Part print with two shaded views. Sizes in mm from the minimum x, y, z corner. A direction names the side the tool comes from. Give positions to 0.01 mm unless a question says otherwise; leave off trailing zeros. Write each loop counter-clockwise with the first axis right and the second up, starting at its lowest first coordinate (ties: lowest second). Pieces come first, ordered by that corner, then holes.
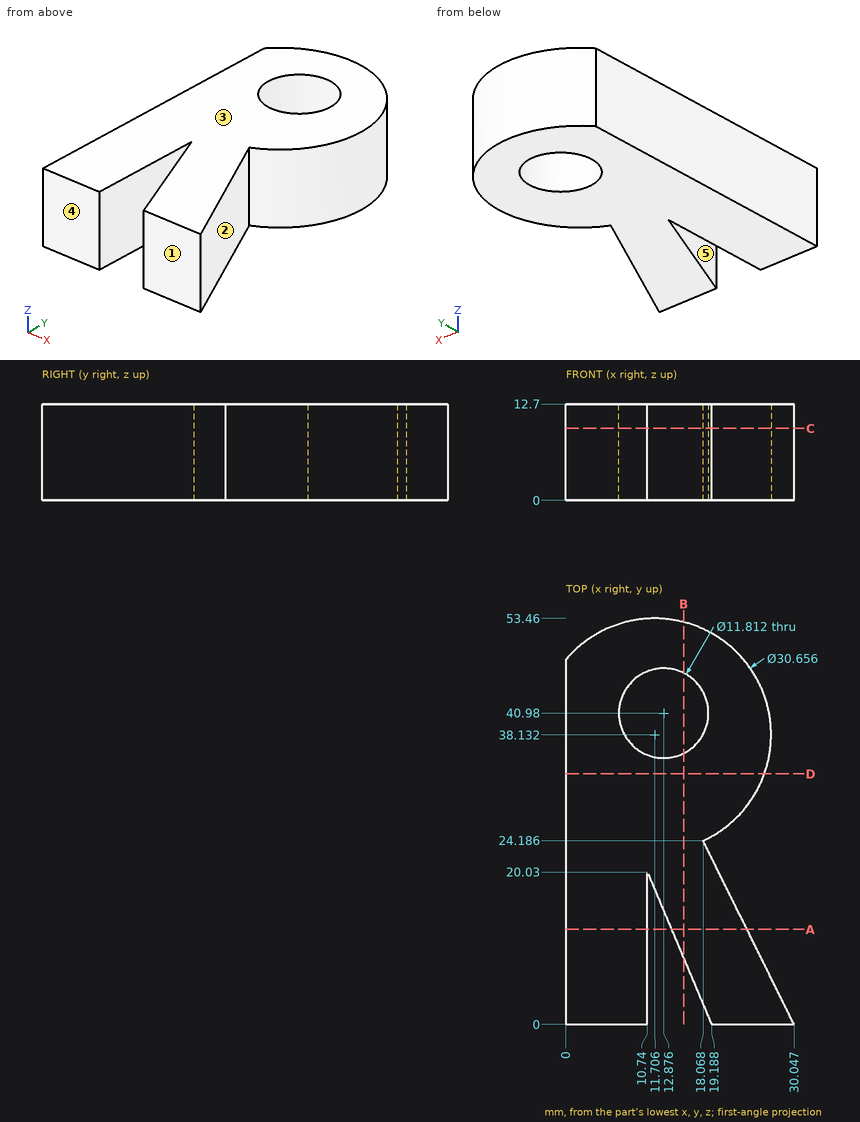
1) Saw through at A-A (y = 12.5). Write the cut outline in (x, z) (1 decimal).
Check result:
outline: (0, 0) - (10.7, 0) - (10.7, 12.7) - (0, 12.7) - close; (13.9, 0) - (23.9, 0) - (23.9, 12.7) - (13.9, 12.7) - close
2) Saw through at B-B (x = 15.5). Write the cut outline in (y, z) (1 decimal).
Check result:
outline: (8.7, 0) - (35.7, 0) - (35.7, 12.7) - (8.7, 12.7) - close; (46.3, 0) - (53, 0) - (53, 12.7) - (46.3, 12.7) - close
3) 3-axis set-ups, long thin cutter, end or side, ignore diameter. For the marked faces 4 and 5: which of +Z, -Z, +X, -X, +Y, -Y reach the whole face in a straight line?
Check result:
face 4: +Z, -Z, +X, -X, -Y
face 5: +Z, -Z, -Y
4) Saw through at D-D (y = 33). Write the cut outline in (x, z), and give its area (3 significant figures).
Check result:
outline: (0, 0) - (26.15, 0) - (26.15, 12.7) - (0, 12.7) - close
area: 332 mm2
5) Saw through at C-C (z = 9.5). Write the cut outline in (x, y) (1 decimal).
Check result:
outline: (0, 0) - (10.7, 0) - (10.7, 20) - (19.2, 0) - (30, 0) - (18.1, 24.2) arc R15.3 ccw (long way) to (0, 48) - close; hole circle Ø11.8 at (12.9, 41)
6) Mould opens along Y. For the marked faces 1, 2 and 3 say: +Y half, -Y half, draft (parallel to the pull), parting line (faces both ways), or undercut.
Check result:
face 1: -Y half
face 2: undercut
face 3: draft
7) Flat gauge pins, fed straight in: P1, Ø2, axis at y = 22.5, z = 4.5, coming from the +X side; P2, Ø5, axis at y = 35, z = 10.5, coming from the +X side; P3, Ø12, axis at x = 26, y = 7, coming from the -Z side; P4, Ø6, axis at x = 5.5, z = 10, coming from the +Y side. Where does each tip first touch, or does it go through?
Check result:
P1: stops at x = 19.4
P2: stops at x = 27.02
P3: stops at z = 0
P4: stops at y = 53.12
8) Drill centre lines: L1, parallel to Y at x = 24, z = 10.25 (1 decimal); L2, parallel to Y at x = 10, z = 3 (1 decimal); L3, parallel to X at y = 18, z = 4.25 (1 decimal). Where is each one in solid material? Low to high.
Check result:
L1: y = 0 to 12.2, 29 to 47.3
L2: y = 0 to 35.8, 46.1 to 53.4
L3: x = 0 to 10.7, 11.6 to 21.1
